For this review, take the finished solid that the model builds, in its own axes (mm). A direction names the side the tool comes from. Round coordinates to 2 decimals unless told otherwise and drop trailing zeros. Order: outer loops, then holes, each group sorted by start corner. A loop starts at its lowest first (then second) coordinate and runs counter-clockwise, first axis right, second up. Notation, with made-up numbers: (84.25, 42) -> (91.25, 42) arc R14 cw to (91.25, 47) -> close; hole circle Ø10 at (11.5, 51.25). An arc over 180 degrees is marked (long way). Answer in a Markdown table with one row per item.
```python
from build123d import *

# Parameters (mm, degrees)
F0_W     = 24.55
F0_H     = 22
F1_DEPTH = 42
F2_SIZE  = 4
F4_D     = 5
F4_DEPTH = 15
F4_TIP   = 1.5021515476


with BuildPart() as f1:
    # F0 (on Right) → F1 (new body)
    with BuildSketch(Plane.YZ):
        with Locations((-12.275, 11)):
            Rectangle(F0_W, F0_H)
    extrude(amount=F1_DEPTH)

    # F2
    f2_edges = [f1.edges().sort_by_distance(p)[0] for p in [
        (21, -24.55, 22),
    ]]
    chamfer(f2_edges, length=F2_SIZE)

    # F4
    with Locations(Plane(origin=(0, 0, 0), x_dir=(1, 0, 0), z_dir=(0, 0, -1))):
        with Locations((32, 12.5), (16, 12.5), (7, 12.5)):
            Hole(F4_D / 2, depth=F4_DEPTH)
            with Locations((0, 0, -(F4_DEPTH + F4_TIP / 2))):  # 118° drill point
                Cone(0, F4_D / 2, F4_TIP, mode=Mode.SUBTRACT)


solid = f1.part
```
Q1. The part is to be moulded in two halves that separate along Y. For faces 3 (the face through (18, -11, 8)), 4 (the face through (0, -12, 11)), 5 (the face through (21, 0, 11)), say which applies: +Y half, -Y half, draft (parallel to the pull), parting line (faces both ways), or undercut.
Answer key:
| item | result |
|---|---|
| face 3 | undercut |
| face 4 | draft |
| face 5 | +Y half |
Q2. Tool access review of faces 1 (the face through (7.54, -10.06, 7.6)), 2 (the face through (21, -24.55, 9)): name each direction out of +Z, -Z, +X, -X, +Y, -Y from which nothing blocks a thin tool from reaching the whole face with its end or side.
Answer key:
| item | result |
|---|---|
| face 1 | -Z |
| face 2 | +Z, -Z, +X, -X, -Y |
Q3. To check wall thickness, follow probe 1 along X at (y, z) = (-12.5, 9.5); probe 2 along Y at (x, z) = (32, 6.5); probe 3 along Y at (x, z) = (32, 15.75). State the ranges of each line that lie inside material, in increasing order.
Answer key:
| item | result |
|---|---|
| probe 1 | x = 0 to 4.5, 9.5 to 13.5, 18.5 to 29.5, 34.5 to 42 |
| probe 2 | y = -24.55 to -15, -10 to 0 |
| probe 3 | y = -24.55 to -13.75, -11.25 to 0 |
Q4. Take a section at A-A, the plane z = 12. Write out the cut boundary in (x, y), then the cut area to 3 significant figures.
Answer key:
| item | result |
|---|---|
| outline | (0, -24.55) -> (42, -24.55) -> (42, 0) -> (0, 0) -> close; hole circle Ø5 at (7, -12.5); hole circle Ø5 at (16, -12.5); hole circle Ø5 at (32, -12.5) |
| area | 972 mm^2 |
